Read the model definition and answer for the solid it produces. Units are mm, in the model's axes. A direction names the side the tool comes from. Coordinates: 2 decimals unless noted, no trailing zeros. Loops run counter-clockwise (first coordinate to the right, second up) from the corner with the lowest first, then second, coordinate; pieces in that order, holes last. Notation, with made-up numbers: (41, 26) -> (69, 26) arc R30 cw to (69, 62) -> close; hole circle Ø2 at (-15.75, -22.75). An arc over 180 degrees is marked (long way). Answer as a JSON object with one key per item and string values. Group by question number.
1) Section B-B, the plane z = 18.75 is taken. Give the vertices of the cut face in (x, y), plus the area to 3 significant figures.
2) Consider probe 1 along X at (y, z) = (116.5, 1.25); probe 2 along Y at (x, z) = (-27, 10.75); probe 3 along Y at (x, z) = (-30, 16.5). Determine where each line is inside the solid, lowest interval first. Write a range as [from, to].
3) Section C-C, the plane y = 140.5 is taken. Give the vertices of the cut face in (x, z).
4) Determine the mould class of faces 1 (the face through (0, 72, 10)), 2 (the face through (-23, 69, 20)), 3 (the face through (-45, 72, 10)) for opening direction X: released by +X, released by -X, zero draft, split by the parting line, or undercut.
5) Which of the six approach directions +Z, -Z, +X, -X, +Y, -Y give full straight-line access (tool end or side, diameter ignored) to faces 4 (the face through (-22.18, 142.65, 3.01)), 5 (the face through (-48.94, 145.27, 8.5))?
6) A flat-ended cylindrical pin translates along its axis: P1, Ø6, axis at y = 36.5, z = 12, coming from the -X side. Find the tip coordinate at first contact, or state that the pin passes through.
7) Section A-A, the plane y = 39 is taken. Give the vertices of the cut face in (x, z).
from build123d import *

# Parameters (mm, degrees)
CROQUIS1_W              = 45
CROQUIS1_H              = 145.5
SALIENTE_EXTRUIR1_DEPTH = 20
REDONDEO1_R             = 10
CROQUIS2_R              = 5
SALIENTE_EXTRUIR2_DEPTH = 8


with BuildPart() as part:
    # Croquis1 → Saliente-Extruir1 (new body)
    with BuildSketch(Plane.XY):
        with Locations((-22.5, 72.75)):
            Rectangle(CROQUIS1_W, CROQUIS1_H)
    extrude(amount=SALIENTE_EXTRUIR1_DEPTH)

    # Redondeo1
    redondeo1_edges = [part.edges().sort_by_distance(p)[0] for p in [
        (-22.5, 145.5, 0),
        (-22.5, 145.5, 20),
    ]]
    fillet(redondeo1_edges, radius=REDONDEO1_R - 0.0001)  # a hair under: the kernel refuses the full size

    # Croquis2 → Saliente-Extruir2 (add)
    with BuildSketch(Plane.ZY.offset(45)):
        with Locations(Location((10, 140.5, 0), (0, 0, 89.99948753))):
            Circle(CROQUIS2_R)
    extrude(amount=SALIENTE_EXTRUIR2_DEPTH)


solid = part.part
Determined:
{
 "1": {"outline": "(-45, 0) -> (0, 0) -> (0, 140.34) -> (-45, 140.34) -> close", "area": "6,320 mm²"},
 "2": {"probe 1": "[-45, 0]", "probe 2": "[0, 145.47]", "probe 3": "[0, 143.1]"},
 "3": {"outline": "(-53, 5) -> (-45, 5) -> (-45, 1.34) -> (0, 1.34) -> (0, 18.66) -> (-45, 18.66) -> (-45, 15) -> (-53, 15) -> close"},
 "4": {"face 1": "released by +X", "face 2": "zero draft", "face 3": "released by -X"},
 "5": {"face 4": "-Z, +X, -X, +Y", "face 5": "-X"},
 "6": {"P1": "x = -45"},
 "7": {"outline": "(-45, 0) -> (0, 0) -> (0, 20) -> (-45, 20) -> close"}
}
